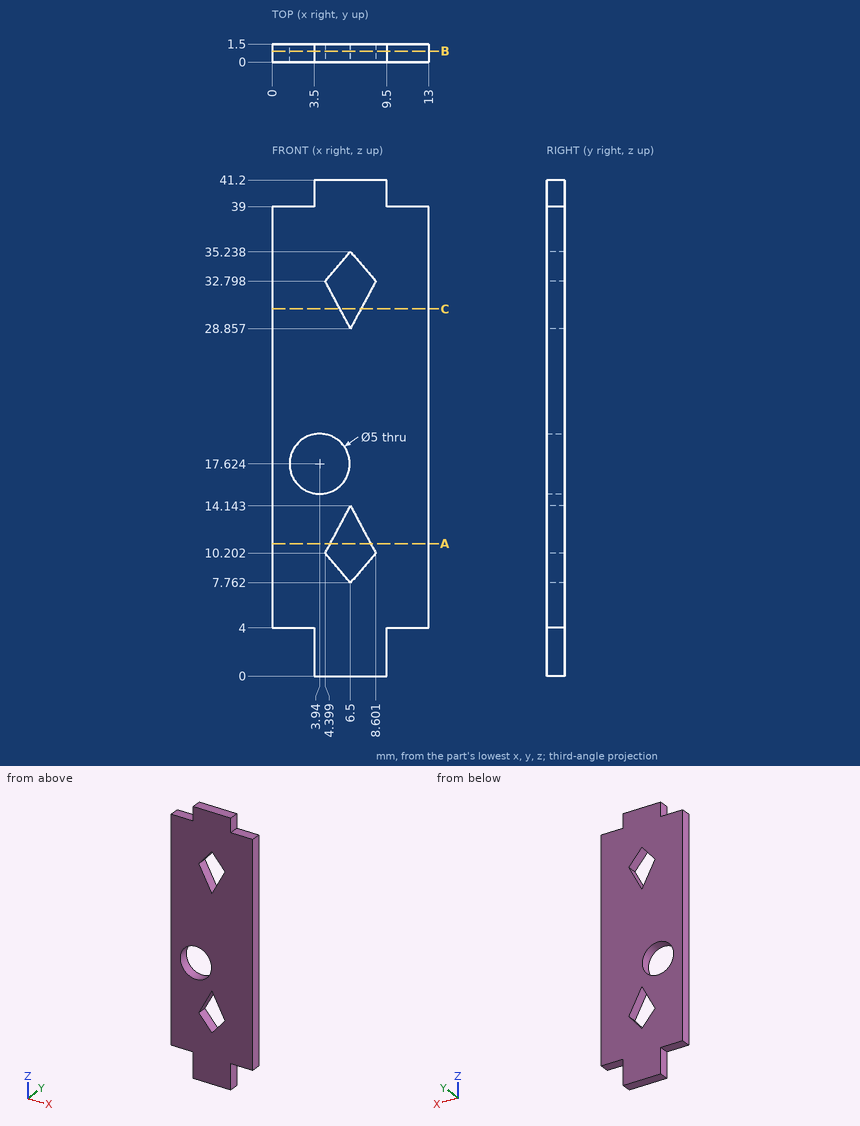
Here's the drawing with two shaded views (mm, measured from the low corner). I have some questions. Round coordinates to 2 decimals unless told otherwise and drop trailing zeros. Loops run counter-clockwise (first coordinate to the right, second up) from the corner with the lowest first, then second, coordinate; pieces in that order, holes last.
1. Suppose I cut it at A-A, the plane z = 11. Please give me the cut outline in (x, y) (1 decimal).
Answers:
outline: (0, 0) - (4.8, 0) - (4.8, 1.5) - (0, 1.5) - close; (8.2, 0) - (13, 0) - (13, 1.5) - (8.2, 1.5) - close
2. If I drill on probe 1 along Z at (x, y) = (7.75, 0.45) (1 decimal); probe 2 along Z at (x, y) = (4.5, 0.7) (1 decimal); probe 3 along Z at (x, y) = (4.75, 1.4) (1 decimal), over which ranges is the centre line in solid material (lowest first)?
Answers:
probe 1: z = 0 to 9.2, 11.8 to 31.2, 33.8 to 41.2
probe 2: z = 0 to 10.1, 10.4 to 15.2, 20.1 to 32.6, 32.9 to 41.2
probe 3: z = 0 to 9.8, 10.9 to 15.3, 20 to 32.1, 33.2 to 41.2
3. Suppose I cut it at B-B, the plane y = 0.9. Please give me the cut outline in (x, z).
Answers:
outline: (0, 4) - (3.5, 4) - (3.5, 0) - (9.5, 0) - (9.5, 4) - (13, 4) - (13, 39) - (9.5, 39) - (9.5, 41.2) - (3.5, 41.2) - (3.5, 39) - (0, 39) - close; hole circle Ø5 at (3.94, 17.62); hole (4.4, 10.2) - (6.5, 7.76) - (8.6, 10.2) - (6.5, 14.14) - close; hole (4.4, 32.8) - (6.5, 28.86) - (8.6, 32.8) - (6.5, 35.24) - close
4. Will these pins go through, and if not, where does the flat tip stop? pin 1 (0.8 mm diameter, centred on x = 1.5, y = 0.5, fed in from -Z); pin 2 (0.8 mm diameter, centred on x = 11, y = 0.5, fed in from +Z).
Answers:
pin 1: stops at z = 4
pin 2: stops at z = 39
5. Suppose I cut it at C-C, the plane z = 30.5. Please give me the cut outline in (x, y) (1 decimal).
Answers:
outline: (0, 0) - (5.6, 0) - (5.6, 1.5) - (0, 1.5) - close; (7.4, 0) - (13, 0) - (13, 1.5) - (7.4, 1.5) - close
